```python
from build123d import *

# Parameters (mm, degrees)
SKETCH1_W                  = 99.441
SKETCH1_H                  = 139.7
EXTRUDE1_DEPTH             = 6.35
SKETCH2_W                  = 66.802
SKETCH2_H                  = 19.05
SKETCH2_W_2                = 26.289
SKETCH2_H_2                = 127
SKETCH2_H_3                = 76.2
CUT_EXTRUDE1_DEPTH         = 6.35
FILLET1_R                  = 6.35
TAP_DRILL_FOR_6_TAP1_D     = 2.7051
TAP_DRILL_FOR_6_TAP1_DEPTH = 12.7
TAP_DRILL_FOR_6_TAP1_TIP   = 0.81269403
TAP_DRILL_FOR_6_TAP2_D     = 2.7051
TAP_DRILL_FOR_6_TAP2_DEPTH = 12.7
TAP_DRILL_FOR_6_TAP2_TIP   = 0.81269403
F_6_CLEARANCE_HOLE1_D      = 3.7973
F_6_CLEARANCE_HOLE1_DEPTH  = 12.7
F_6_CLEARANCE_HOLE1_TIP    = 1.140824014
SKETCH6_W                  = 19.05
SKETCH6_H                  = 22.225
EXTRUDE2_DEPTH             = 6.35
FILLET2_R                  = 6.35
F_6_CLEARANCE_HOLE2_D      = 3.7973
F_6_CLEARANCE_HOLE2_DEPTH  = 12.7
F_6_CLEARANCE_HOLE2_TIP    = 1.140824014


with BuildPart() as part:
    # Sketch1 → Extrude1 (new body)
    with BuildSketch(Plane(origin=(0, 0, 0), x_dir=(1, 0, 0), z_dir=(0, 1, 0))):
        Rectangle(SKETCH1_W, SKETCH1_H)
    extrude(amount=EXTRUDE1_DEPTH)

    # Sketch2 → Cut-Extrude1 (cut)
    with BuildSketch(Plane(origin=(0, 6.35, 0), x_dir=(-1, 0, 0), z_dir=(0, 1, 0))):
        with Locations((16.3195, -60.325)):
            Rectangle(SKETCH2_W, SKETCH2_H)
        with Locations((16.3195, 60.325)):
            Rectangle(SKETCH2_W, SKETCH2_H)
        with Locations((-36.576, 0)):
            Rectangle(SKETCH2_W_2, SKETCH2_H_2)
        with Locations((16.3195, 0)):
            Rectangle(SKETCH2_W, SKETCH2_H_3)
    extrude(amount=-CUT_EXTRUDE1_DEPTH, mode=Mode.SUBTRACT)

    # Fillet1
    fillet1_edges = [part.edges().sort_by_distance(p)[0] for p in [
        (17.0815, 3.175, -50.8),
        (17.0815, 3.175, 50.8),
        (23.4315, 3.175, 63.5),
        (23.4315, 3.175, -63.5),
        (17.0815, 3.175, -38.1),
        (17.0815, 3.175, 38.1),
    ]]
    fillet(fillet1_edges, radius=FILLET1_R)

    # Tap Drill for #6 Tap1
    with Locations(Plane(origin=(-49.7205, 3.175, -44.45), x_dir=(0, 0, -1), z_dir=(-1, 0, 0))):
        with Locations((0, 0), (-88.9, 0)):
            Hole(TAP_DRILL_FOR_6_TAP1_D / 2, depth=TAP_DRILL_FOR_6_TAP1_DEPTH)
            with Locations((0, 0, -(TAP_DRILL_FOR_6_TAP1_DEPTH + TAP_DRILL_FOR_6_TAP1_TIP / 2))):  # 118° drill point
                Cone(0, TAP_DRILL_FOR_6_TAP1_D / 2, TAP_DRILL_FOR_6_TAP1_TIP, mode=Mode.SUBTRACT)

    # Tap Drill for #6 Tap2
    with Locations(Plane(origin=(49.7205, 3.175, -66.675), x_dir=(0, 0, 1), z_dir=(1, 0, 0))):
        with Locations((0, 0), (133.35, 0)):
            Hole(TAP_DRILL_FOR_6_TAP2_D / 2, depth=TAP_DRILL_FOR_6_TAP2_DEPTH)
            with Locations((0, 0, -(TAP_DRILL_FOR_6_TAP2_DEPTH + TAP_DRILL_FOR_6_TAP2_TIP / 2))):  # 118° drill point
                Cone(0, TAP_DRILL_FOR_6_TAP2_D / 2, TAP_DRILL_FOR_6_TAP2_TIP, mode=Mode.SUBTRACT)

    # #6 Clearance Hole1
    with Locations(Plane(origin=(20.2565, 0, 6.35), x_dir=(0, 0, -1), z_dir=(0, -1, 0))):
        with Locations((0, 0), (12.7, 0)):
            Hole(F_6_CLEARANCE_HOLE1_D / 2, depth=F_6_CLEARANCE_HOLE1_DEPTH)
            with Locations((0, 0, -(F_6_CLEARANCE_HOLE1_DEPTH + F_6_CLEARANCE_HOLE1_TIP / 2))):  # 118° drill point
                Cone(0, F_6_CLEARANCE_HOLE1_D / 2, F_6_CLEARANCE_HOLE1_TIP, mode=Mode.SUBTRACT)

    # Sketch6 → Extrude2 (add)
    with BuildSketch(Plane.XZ):
        with Locations((-14.7955, 61.9125)):
            Rectangle(SKETCH6_W, SKETCH6_H)
        with Locations((-14.7955, -61.9125)):
            Rectangle(SKETCH6_W, SKETCH6_H)
    extrude(amount=-EXTRUDE2_DEPTH)

    # Fillet2
    fillet2_edges = [part.edges().sort_by_distance(p)[0] for p in [
        (-5.2705, 3.175, 50.8),
        (-24.3205, 3.175, 50.8),
        (-5.2705, 3.175, -50.8),
        (-24.3205, 3.175, -50.8),
    ]]
    fillet(fillet2_edges, radius=FILLET2_R)

    # #6 Clearance Hole2
    with Locations(Plane(origin=(-8.4455, 0, 69.85), x_dir=(0, 0, -1), z_dir=(0, -1, 0))):
        with Locations((0, 0), (139.7, -12.7), (0, -12.7), (139.7, 0)):
            Hole(F_6_CLEARANCE_HOLE2_D / 2, depth=F_6_CLEARANCE_HOLE2_DEPTH)
            with Locations((0, 0, -(F_6_CLEARANCE_HOLE2_DEPTH + F_6_CLEARANCE_HOLE2_TIP / 2))):  # 118° drill point
                Cone(0, F_6_CLEARANCE_HOLE2_D / 2, F_6_CLEARANCE_HOLE2_TIP, mode=Mode.SUBTRACT)


solid = part.part
```
Could you check a few things on this model? Use its own coordinates, in mm. A direction names the side the tool comes from. Round coordinates to 2 decimals unless told otherwise and drop trailing zeros. Write each loop counter-clockwise with the first axis right and the second up, starting at its lowest first coordinate (ties: lowest second). Pieces come first, ordered by that corner, then holes. Notation, with made-up numbers: M 78.25,53.5 L 107.25,53.5 A28 cw 107.25,83.5 Z; hole C -37.5,-18.5 d5. An arc over 180 degrees is marked long. Answer in a Markdown table with one row per item. Add a question column.
Q1. Imagine slicing it at B-B (z = 6.35). Please give me the cut outline in (x, y).
Q2. Imagine slicing it at C-C (z = 60.5). Please give me the cut outline in (x, y), then the cut area to 3 significant figures.
Q3. If I drill on line 1 (Z direction, x = -44, y = 5); line 2 (Z direction, x = 33, y = 2.25); line 3 (Z direction, x = -10, y = 5.5) (3 decimals), over which ranges is the centre line in solid material (lowest first)? Write a range as from..to.
Q4. Imagine slicing it at A-A (x = 44). Please give me the cut outline in (y, z) (3 decimals), then the cut area to 3 significant figures.
Q5. On a 3-axis mill with a long thin cutter (end or side, diameter ignored), from which of +Z, -Z, +X, -X, +Y, -Y can I reach the whole of each face in a straight line? I mean faces 1 (the flat face through (-5.27, 3, 65)), 2 (the flat face through (-40, 3, 50.8)), 3 (the cylindrical face through (15.17, 3.13, 36.29)), 4 (the flat face through (-5.27, 3, -65)), 5 (the conical face through (-36.35, 3.32, 44.64)). Say none if no direction works.
Q6. Imagine slicing it at D-D (z = -49). Please give me the cut outline in (x, y).
Q7. Will these pins go through, and if not, where does the flat tip stop? pin 1 Ø3 at (y, z) = (3.5, -62.5) entering from -X; pin 2 Ø1 at (y, z) = (4, 44) entering from +X; pin 3 Ø3 at (x, y) = (-42, 2) entering from +Z; pin 4 Ø3.5 at (x, z) = (-21.15, -69.85) entering from -Y (3 decimals).
Q8. If we mould it in two halves opening along X, with no side actions, what happens to faces 6 (the flat face through (-19, 3, -38.1)), 7 (the cylindrical face through (15.17, 3.13, -52.61)), 8 (the flat face through (-24.321, 3, -65)), 9 (the cylindrical face through (18.403, 3.219, 5.938))? For each: +X half, -X half, draft (parallel to the pull), parting line (faces both ways), or undercut.
Values:
| question | item | result |
|---|---|---|
| 1 | outline | M 17.08,0 L 18.36,0 L 18.36,6.35 L 17.08,6.35 Z; M 22.16,0 L 23.43,0 L 23.43,6.35 L 22.16,6.35 Z |
| 2 | outline | M -24.32,0 L -5.27,0 L -5.27,6.35 L -24.32,6.35 Z; M 17.08,0 L 24.39,0 L 24.39,6.35 L 17.08,6.35 Z |
| 2 | area | 167 mm^2 |
| 3 | line 1 | -50.8..-38.1, 38.1..50.8 |
| 3 | line 2 | -69.85..-63.5, 63.5..69.85 |
| 3 | line 3 | -73.025..-70.94, -68.76..-38.1, 38.1..68.76, 70.94..73.025 |
| 4 | outline | M 0,-69.85 L 6.35,-69.85 L 6.35,-63.5 L 0,-63.5 Z; M 0,63.5 L 6.35,63.5 L 6.35,69.85 L 0,69.85 Z; hole C 3.175,-66.675 d2.705; hole C 3.175,66.675 d2.705 |
| 4 | area | 69.2 mm^2 |
| 5 | face 1 | +Z, +Y, -Y |
| 5 | face 2 | +Z, -X, +Y, -Y |
| 5 | face 3 | -X, +Y, -Y |
| 5 | face 4 | -Z, +Y, -Y |
| 5 | face 5 | -X |
| 6 | outline | M -49.72,0 L 23.43,0 L 23.43,6.35 L -49.72,6.35 Z |
| 7 | pin 1 | x = -24.32 |
| 7 | pin 2 | x = 23.43 |
| 7 | pin 3 | z = 50.8 |
| 7 | pin 4 | through |
| 8 | face 6 | draft |
| 8 | face 7 | undercut |
| 8 | face 8 | -X half |
| 8 | face 9 | undercut |
